from build123d import *

# Parameters (mm, degrees)
BOSS_EXTRUDE1_DEPTH = 4


with BuildPart() as part:
    # Sketch1 → Boss-Extrude1 (new body)
    with BuildSketch(Plane.XY):
        with BuildLine():
            Line((30.862718171, 33.494054131), (69.862718171, 33.494054131))
            Line((69.862718171, 33.494054131), (69.862718171, 8.494054131))
            Line((69.862718171, 8.494054131), (30.862718171, 8.494054131))
            Line((30.862718171, 8.494054131), (30.862718171, -9.005945869))
            Line((30.862718171, -9.005945869), (-39.137281829, -9.005945869))
            Line((-39.137281829, -9.005945869), (-39.137281829, 7.037446143))
            ThreePointArc((-39.137281829, 7.037446143), (-30.320886371, 19.996051834), (-17.137281829, 28.472304637))
            Line((-17.137281829, 28.472304637), (-17.137281829, 50.994054131))
            Line((-17.137281829, 50.994054131), (30.862718171, 50.994054131))
            Line((30.862718171, 50.994054131), (30.862718171, 33.494054131))
        make_face()
        with BuildLine():
            Line((-4.137281829, 38.994054131), (-4.137281829, -1.005945869))
            ThreePointArc((-4.137281829, -1.005945869), (-1.637281829, -3.505945869), (0.862718171, -1.005945869))
            Line((0.862718171, -1.005945869), (0.862718171, 38.994054131))
            ThreePointArc((0.862718171, 38.994054131), (-1.637281829, 41.494054131), (-4.137281829, 38.994054131))
        make_face(mode=Mode.SUBTRACT)
        with BuildLine():
            Line((-12.137281829, 33.312431903), (-12.137281829, 2.809827896))
            ThreePointArc((-12.137281829, 2.809827896), (-9.637281829, 0.309827896), (-7.137281829, 2.809827896))
            Line((-7.137281829, 2.809827896), (-7.137281829, 33.312431903))
            ThreePointArc((-7.137281829, 33.312431903), (-9.637281829, 35.812431903), (-12.137281829, 33.312431903))
        make_face(mode=Mode.SUBTRACT)
        with BuildLine():
            Line((-15.137281829, 23.861283589), (-15.137281829, 7.683449462))
            ThreePointArc((-15.137281829, 7.683449462), (-17.637281829, 5.183449462), (-20.137281829, 7.683449462))
            Line((-20.137281829, 7.683449462), (-20.137281829, 23.861283589))
            ThreePointArc((-20.137281829, 23.861283589), (-17.637281829, 26.361283589), (-15.137281829, 23.861283589))
        make_face(mode=Mode.SUBTRACT)
        with BuildLine():
            Line((3.862718171, 30.994054131), (3.862718171, 2.647434443))
            ThreePointArc((3.862718171, 2.647434443), (6.362718171, 0.147434443), (8.862718171, 2.647434443))
            Line((8.862718171, 2.647434443), (8.862718171, 30.994054131))
            ThreePointArc((8.862718171, 30.994054131), (6.362718171, 33.494054131), (3.862718171, 30.994054131))
        make_face(mode=Mode.SUBTRACT)
        with BuildLine():
            Line((11.862718171, 22.048271006), (11.862718171, 5.538473012))
            ThreePointArc((11.862718171, 5.538473012), (14.362718171, 3.038473012), (16.862718171, 5.538473012))
            Line((16.862718171, 5.538473012), (16.862718171, 22.048271006))
            ThreePointArc((16.862718171, 22.048271006), (14.362718171, 24.548271006), (11.862718171, 22.048271006))
        make_face(mode=Mode.SUBTRACT)
    extrude(amount=BOSS_EXTRUDE1_DEPTH)


solid = part.part
Build history of the part. All positions in model axes, mm. A direction names the side the tool comes from. Round coordinates to 2 decimals unless told otherwise and drop trailing zeros. Order: outer loops, then holes, each group sorted by start corner. A loop starts at its lowest first (then second) coordinate and runs counter-clockwise, first axis right, second up. Notation, with made-up numbers: M 0.25,15.5 L 18.25,15.5 A10 cw 18.25,27.5 Z; hole C 62,42 d11. An arc over 180 degrees is marked long. Use CSV: the item, a comma, the result in double quotes. Start each with the question number.
(1) Cut at B-B on y = 19. List the corners of the cut face in (x, z), then the cut area to 3 significant figures.
(2) Cut at A-A on z = 2.35. State how many separate pieces and enclosed holes the cut face has, then the cut area to 3 significant figures.
(3) Tool access for faces 4 (the face through (69.863, 21, 2)), 5 (the face through (11.863, 14, 2)): list every direction of +Z, -Z, +X, -X, +Y, -Y with a clear straight run to the whole face (end or side of a thin tool).
(4) Drill centre lines: probe 1 along X at (y, z) = (29, 0.2); probe 2 along X at (y, z) = (0, 1.35); probe 3 along X at (y, z) = (23, 1.4). Where is each one in solid material? Low to high.
(5) Flat gauge pins, fed straight in: P1, Ø3, axis at x = 41, y = 27, coming from the -Z side; P2, Ø1.2, axis at x = 46.5, z = 2, coming from the +Y side. Where does each tip first touch, or does it go through?
(6) Cut at C-C on x = 42. List the corners of the cut face in (y, z), then the cut area to 3 significant figures.
(7) Mould opens along X. For faces 1 (the face through (30.863, 42, 2)), 2 (the face through (-9.58, 35.81, 1.97)), 3 (the face through (51, 8.494, 2)) say: +X half, -X half, draft (parallel to the pull), parting line (faces both ways), or undercut.
(8) Cut at D-D on y = 11. List the corners of the cut face in (x, z), then the cut area to 3 significant figures.
Findings:
1,outline,"M -31.31,0 L -20.14,0 L -20.14,4 L -31.31,4 Z; M -15.14,0 L -12.14,0 L -12.14,4 L -15.14,4 Z; M -7.14,0 L -4.14,0 L -4.14,4 L -7.14,4 Z; M 0.86,0 L 3.86,0 L 3.86,4 L 0.86,4 Z; M 8.86,0 L 11.86,0 L 11.86,4 L 8.86,4 Z; M 16.86,0 L 69.86,0 L 69.86,4 L 16.86,4 Z"
1,area,"305 mm^2"
2,separate pieces,"1"
2,enclosed holes,"5"
2,area,"3,750 mm^2"
3,face 4,"+Z, -Z, +X, +Y, -Y"
3,face 5,"+Z, -Z"
4,probe 1,"x = -17.14 to -12.14, -7.14 to -4.14, 0.86 to 3.86, 8.86 to 69.86"
4,probe 2,"x = -39.14 to -4.14, 0.86 to 30.86"
4,probe 3,"x = -26.85 to -20.14, -15.14 to -12.14, -7.14 to -4.14, 0.86 to 3.86, 8.86 to 12.05, 16.67 to 69.86"
5,P1,"stops at z = 0"
5,P2,"stops at y = 33.49"
6,outline,"M 8.49,0 L 33.49,0 L 33.49,4 L 8.49,4 Z"
6,area,"100 mm^2"
7,face 1,"+X half"
7,face 2,"undercut"
7,face 3,"draft"
8,outline,"M -37.21,0 L -20.14,0 L -20.14,4 L -37.21,4 Z; M -15.14,0 L -12.14,0 L -12.14,4 L -15.14,4 Z; M -7.14,0 L -4.14,0 L -4.14,4 L -7.14,4 Z; M 0.86,0 L 3.86,0 L 3.86,4 L 0.86,4 Z; M 8.86,0 L 11.86,0 L 11.86,4 L 8.86,4 Z; M 16.86,0 L 69.86,0 L 69.86,4 L 16.86,4 Z"
8,area,"328 mm^2"
